Part print with two shaded views. Sizes in mm from the minimum x, y, z corner. Round coordinates to 2 decimals unless told otherwise and drop trailing zeros. Order: outer loops, then holes, each group sorted by start corner. A loop starts at its lowest first (then second) coordinate and runs counter-clockwise, first axis right, second up. Notation, with made-up numbers: (45.5, 37.25) -> (87.5, 37.25) arc R31 ccw to (87.5, 61.25) -> close; hole circle Ø3 at (-6.5, -5). An arc over 180 degrees is marked (long way). Answer as a JSON object with one key per item and string values.
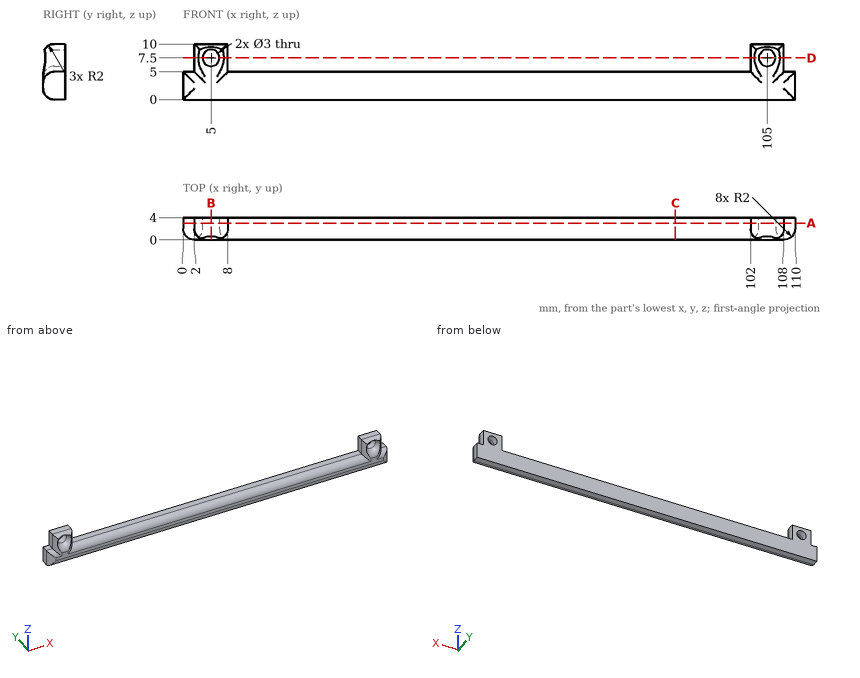
1) Cut at D-D, the plane z = 7.5. Give the cut face in (x, y), plus the area to 3 significant figures.
Checked values:
{"outline": "(2, 2) arc R2 ccw to (2.75, 0.44) arc R2 ccw to (3.5, 2) -> (3.5, 4) -> (2, 4) -> close; (6.5, 2) arc R2 ccw to (7.25, 0.44) arc R2 ccw to (8, 2) -> (8, 4) -> (6.5, 4) -> close; (102, 2) arc R2 ccw to (102.75, 0.44) arc R2 ccw to (103.5, 2) -> (103.5, 4) -> (102, 4) -> close; (106.5, 2) arc R2 ccw to (107.25, 0.44) arc R2 ccw to (108, 2) -> (108, 4) -> (106.5, 4) -> close", "area": "18.5 mm²"}
2) Cut at A-A, the plane y = 3. Give the cut face in (x, z), plus the area to 3 significant figures.
Checked values:
{"outline": "(0, 0) -> (110, 0) -> (110, 5) -> (108, 5) -> (108, 10) -> (102, 10) -> (102, 5) -> (8, 5) -> (8, 10) -> (2, 10) -> (2, 5) -> (0, 5) -> close; hole circle Ø3 at (5, 7.5); hole circle Ø3 at (105, 7.5)", "area": "596 mm²"}
3) Flat gauge pins, fed straight in: pin 1 Ø5 at (x, z) = (89, 8) entering from +Y; pin 2 Ø2 at (y, z) = (2, 8) entering from -X; pin 3 Ø2 at (y, z) = (3.5, 6.5) entering from +X; pin 4 Ø4 at (x, z) = (76, 6.5) entering from -Y. Where does each tip first touch, or does it go through?
Checked values:
{"pin 1": "passes through", "pin 2": "stops at x = 2", "pin 3": "stops at x = 108", "pin 4": "stops at y = 0.68"}
4) Cut at B-B, the plane x = 5. Give the cut face in (y, z), plus the area to 3 significant figures.
Checked values:
{"outline": "(0, 2) arc R2 ccw to (2, 0) -> (4, 0) -> (4, 6) -> (2, 6) arc R2 ccw to (0, 4) -> close; (0.68, 9.5) arc R2 ccw to (2, 9) -> (4, 9) -> (4, 10) -> (2, 10) arc R2 ccw to start", "area": "25.2 mm²"}
5) Probe L1, parallel to X at y = 1.5, z = 8; L2, parallel to Z at x = 105, y = 2.8; L3, parallel to X at y = 1.5, z = 6.5. List the from-to ranges inside material, lowest first. Write a range as from..to.
Checked values:
{"L1": "x = 2.06..3.52, 6.48..7.94, 102.06..103.52, 106.48..107.94", "L2": "z = 0..6, 9..10", "L3": "x = 2.06..3.8, 6.2..7.94, 102.06..103.8, 106.2..107.94"}
6) Cut at C-C, the plane x = 88.5. Give the cut face in (y, z), plus the area to 3 significant figures.
Checked values:
{"outline": "(0, 2) arc R2 ccw to (2, 0) -> (4, 0) -> (4, 5) -> (2, 5) arc R2 ccw to (0, 3) -> close", "area": "18.3 mm²"}
